```python
from build123d import *

# Parameters (mm, degrees)
SKETCH_1_W          = 37
SKETCH_1_H          = 63
EXTRUDE_1_DEPTH     = 16
FILLET_1_R          = 1
CUT_EXTRUDE_START   = 16
SKETCH_1_9_W        = 7.2
SKETCH_1_9_H        = 3.2
CUT_EXTRUDE_1_DEPTH = 2
EXTRUDE_START       = 14
SKETCH_1_10_W       = 3.5
SKETCH_1_10_H       = 3
EXTRUDE_2_DEPTH     = 2.5


with BuildPart() as part:
    # 草图1 → 凸台-拉伸1 (new body)
    with BuildSketch(Plane(origin=(0, 0, 0), x_dir=(1, 0, 0), z_dir=(0, 1, 0))):
        Rectangle(SKETCH_1_W, SKETCH_1_H)
    extrude(amount=EXTRUDE_1_DEPTH)

    # 圆角1
    fillet_1_edges = [part.edges().sort_by_distance(p)[0] for p in [
        (0, 16, -31.5),
        (-18.5, 16, 0),
        (0, 16, 31.5),
        (-18.5, 0, 0),
        (0, 0, -31.5),
        (18.5, 0, 0),
        (0, 0, 31.5),
        (-18.5, 8, 31.5),
        (-18.5, 8, -31.5),
        (18.5, 8, -31.5),
        (18.5, 8, 31.5),
        (18.5, 16, 0),
    ]]
    fillet(fillet_1_edges, radius=FILLET_1_R)

    # 草图1<9> → 切除-拉伸1 (cut)
    with BuildSketch(Plane(origin=(0, 0, 0), x_dir=(1, 0, 0), z_dir=(0, 1, 0)).offset(CUT_EXTRUDE_START)):
        with Locations((6, 25)):
            Rectangle(SKETCH_1_9_W, SKETCH_1_9_H)
    extrude(amount=-CUT_EXTRUDE_1_DEPTH, mode=Mode.SUBTRACT)

    # 草图1<10> → 凸台-拉伸2 (add)
    with BuildSketch(Plane(origin=(0, 0, 0), x_dir=(1, 0, 0), z_dir=(0, 1, 0)).offset(EXTRUDE_START)):
        with Locations((4.25, 25)):
            Rectangle(SKETCH_1_10_W, SKETCH_1_10_H)
    extrude(amount=EXTRUDE_2_DEPTH)


solid = part.part
```
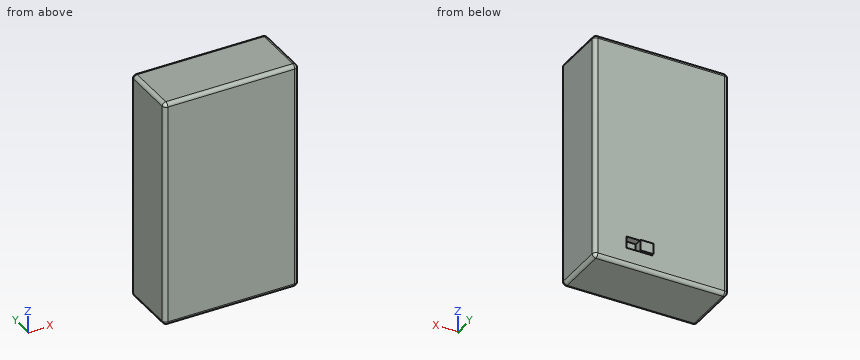
CAD build for the part. Positions are in the model's coordinates, mm. Give positions to 0.01 mm unless a question says otherwise; leave off trailing zeros. Loops run counter-clockwise (first coordinate to the right, second up) from the corner with the lowest first, then second, coordinate; pieces in that order, holes last. Notation, with made-up numbers: (59.5, 59) - (70.5, 59) arc R18 ccw to (70.5, 67) - close; hole circle Ø9 at (62.5, 87). An arc over 180 degrees is marked (long way). Put each result on its own line as item: value.
Q1. Flat gauge pins, fed straight in: pin 1 (1.2 mm diameter, centred on y = 15.5, z = -25, fed in from +X); pin 2 (0.6 mm diameter, centred on x = 4.5, y = 15.5, fed in from +Z); pin 3 (17.5 mm diameter, centred on x = 1, z = 14, fed in from +Y). Where does each tip first touch, or does it go through?
Filled in:
pin 1: stops at x = 18.5
pin 2: stops at z = 31.48
pin 3: stops at y = 16
Q2. Slice it at B-B (x = 4.5). Give the cut face in (y, z).
Filled in:
outline: (0, -30.5) arc R1 ccw to (1, -31.5) - (15, -31.5) arc R1 ccw to (16, -30.5) - (16, -26.6) - (14, -26.6) - (14, -26.5) - (16.5, -26.5) - (16.5, -23.5) - (14, -23.5) - (14, -23.4) - (16, -23.4) - (16, 30.5) arc R1 ccw to (15, 31.5) - (1, 31.5) arc R1 ccw to (0, 30.5) - close
Q3. Probe line 1 along Y through (x, z) = (1.5, 23); line 2 along Z through (x, y) = (-10.5, 15.75). List the from-to ranges inside material, lowest first.
Filled in:
line 1: y = 0 to 16
line 2: z = -31.16 to 31.16
Q4. Slice it at C-C (x = 12.5). Give the cut face in (y, z), plus the area to 3 significant figures.
Filled in:
outline: (0, -30.5) arc R1 ccw to (1, -31.5) - (15, -31.5) arc R1 ccw to (16, -30.5) - (16, 30.5) arc R1 ccw to (15, 31.5) - (1, 31.5) arc R1 ccw to (0, 30.5) - close
area: 1,010 mm²
Q5. Slice it at A-A (z = 15). Give the cut face in (x, y).
Filled in:
outline: (-18.5, 1) arc R1 ccw to (-17.5, 0) - (17.5, 0) arc R1 ccw to (18.5, 1) - (18.5, 15) arc R1 ccw to (17.5, 16) - (-17.5, 16) arc R1 ccw to (-18.5, 15) - close
